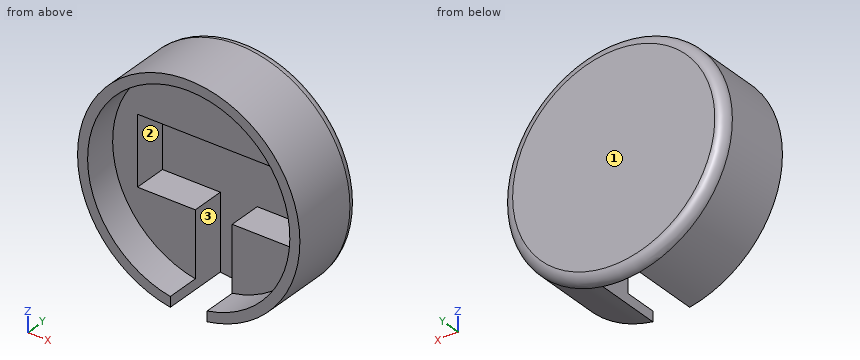
from build123d import *

# Parameters (mm, degrees)
SKETCH1_R           = 33.15
BOSS_EXTRUDE1_DEPTH = 23
SHELL1_T            = -3
BOSS_EXTRUDE2_START = 10
BOSS_EXTRUDE2_DEPTH = 10
CUT_EXTRUDE1_DEPTH  = 20


with BuildPart() as part:
    # Sketch1 → Boss-Extrude1 (new body)
    with BuildSketch(Plane(origin=(0, 0, 0), x_dir=(1, 0, 0), z_dir=(0, 1, 0))):
        with Locations(Location((0, 0, 0), (0, 0, 270))):
            Circle(SKETCH1_R)
    extrude(amount=BOSS_EXTRUDE1_DEPTH)

    # Shell1
    shell1_openings = [part.faces().sort_by_distance(p)[0] for p in [
        (0, 0, 0),
    ]]
    offset(amount=SHELL1_T, openings=shell1_openings, kind=Kind.INTERSECTION)

    # Sketch2 → Boss-Extrude2 (add)
    with BuildSketch(Plane.XZ.offset(-20).offset(BOSS_EXTRUDE2_START)):
        with BuildLine():
            Line((-5.5, -29.64409722), (-5.5, -10.25))
            Line((-5.5, -10.25), (-22.75, -10.25))
            Line((-22.75, -10.25), (-22.75, 10.25))
            Line((-22.75, 10.25), (22.75, 10.25))
            Line((22.75, 10.25), (22.75, -10.25))
            Line((22.75, -10.25), (5.5, -10.25))
            Line((5.5, -10.25), (5.5, -29.64409722))
            ThreePointArc((5.5, -29.64409722), (23.182401731, -19.276896794), (30.15, 0))
            ThreePointArc((30.15, 0), (-19.276896794, 23.182401731), (-5.5, -29.64409722))
        make_face()
    extrude(amount=-BOSS_EXTRUDE2_DEPTH)

    # Sketch3 → Cut-Extrude1 (cut)
    with BuildSketch(Plane.XZ):
        with BuildLine():
            Line((-5.5, -29.64409722), (-5.5, -32.69055674))
            ThreePointArc((-5.5, -32.69055674), (0, -33.15), (5.5, -32.69055674))
            Line((5.5, -32.69055674), (5.5, -29.64409722))
            ThreePointArc((5.5, -29.64409722), (0, -30.15), (-5.5, -29.64409722))
        make_face()
    extrude(amount=-CUT_EXTRUDE1_DEPTH, mode=Mode.SUBTRACT)

    # Fillet1: read off the stored shape, not the designer's step
    # Fillet1 outline → Fillet1 (revolve, cut)
    with BuildSketch(Plane.XY):
        with BuildLine():
            ThreePointArc((30.15, 23), (32.271320344, 22.121320344), (33.15, 20))
            Line((33.15, 20), (33.15, 23))
            Line((33.15, 23), (30.15, 23))
        make_face()
    revolve(axis=Axis((0, 0, 0), (0, 1, 0)), mode=Mode.SUBTRACT)


solid = part.part
Build history of the part. All positions in model axes, mm. Face numbers are marked on the shaded views. A direction names the side the tool comes from. Round coordinates to 2 decimals unless told otherwise and drop trailing zeros. Loops run counter-clockwise (first coordinate to the right, second up) from the corner with the lowest first, then second, coordinate; pieces in that order, holes last. Notation, with made-up numbers: (-14.5, 87) -> (10.5, 87) arc R16 cw to (10.5, 108) -> close; hole circle Ø9 at (75, 6). An arc over 180 degrees is marked (long way). One line per item, written item: value. Start each with the question number.
Q1. Cut at A-A on x = 0. List the corners of the cut face in (y, z).
Q2. Probe line 1 along X through (y, z) = (8, 0); line 2 along Y through (x, z) = (-8, -5.5); line 3 along Y through (x, z) = (-4.5, 15.5). List the from-to ranges inside material, lowest first.
Q3. Cut at C-C on y = 7. List the corners of the cut face in (x, z), plus the area to 3 significant figures.
Q4. Drop flat-ended pins along their axis: pin 1 Ø10 at (x, y) = (-6.5, 18.5) entering from +Z; pin 2 Ø3 at (x, y) = (-15, 14) entering from +Z; pin 3 Ø6 at (y, z) = (7, 15) entering from -X. Give the stop position or say it passes through.
Q5. Cut at B-B on z = 0. List the corners of the cut face in (x, y), plus the area to 3 significant figures.
Q6. 3-axis set-ups, long thin cutter, end or side, ignore diameter. For the marked faces 1, 2 and 3: which of +Z, -Z, +X, -X, +Y, -Y reach the whole face in a straight line?
Computed:
1. outline: (0, 30.15) -> (10, 30.15) -> (10, 10.25) -> (20, 10.25) -> (20, -33.15) arc R3 ccw to (23, -30.15) -> (23, 30.15) arc R3 ccw to (20, 33.15) -> (0, 33.15) -> close
2. line 1: -33.15 to -30.15, 30.15 to 33.15
2. line 2: 20 to 23
2. line 3: 10 to 23
3. outline: (-5.5, -32.69) -> (-5.5, -29.64) arc R30.15 cw (long way) to (5.5, -29.64) -> (5.5, -32.69) arc R33.15 ccw (long way) to start
3. area: 563 mm²
4. pin 1: z = 33.12
4. pin 2: z = 30.28
4. pin 3: x = -30.9
5. outline: (-33.15, 0) -> (-30.15, 0) -> (-30.15, 10) -> (-22.75, 10) -> (-22.75, 20) -> (22.75, 20) -> (22.75, 10) -> (30.15, 10) -> (30.15, 0) -> (33.15, 0) -> (33.15, 20) arc R3 ccw to (30.15, 23) -> (-30.15, 23) arc R3 ccw to (-33.15, 20) -> close
5. area: 463 mm²
6. face 1: +Z, -Z, +X, -X, +Y
6. face 2: -Y
6. face 3: -Z, -Y
